For this review, use the dimensioned drawing (mm, ordinates from the lowest corner) and the shaded views. A direction names the side the tool comes from. Round coordinates to 2 decimals unless told otherwise and drop trailing zeros. Loops run counter-clockwise (first coordinate to the right, second up) from the corner with the lowest first, then second, coordinate; pieces in that order, holes last. Notation, with made-up numbers: M -39.75,-37 L -14.75,-37 A20 ccw -14.75,-11 Z; hole C 64,68 d10. An arc over 180 degrees is marked long. One line per item, written item: value. Start each with the question number.
Item 1: For the marked faces 1 and 2, list the 3-axis set-ups (+Z, -Z, +X, -X, +Y, -Y) from which the entire face can be reached by the end or side of a thin tool; tool diameter is ignored.
Item 2: We need section A-A (y = 12.5). Write out the cut boundary in (x, z), then the cut area to 3 significant figures.
Item 3: For line 1 along Z through (x, y) = (10.25, 12.75); line 2 along Z through (x, y) = (12.5, 20.5); line 3 along X through (y, z) = (17.5, 8.5), list the stretches that pass through material, from the lowest coordinate up.
Item 4: We need section C-C (z = 13.5). Write out the cut boundary in (x, y).
Item 5: We need section B-B (z = 31). Write out the cut boundary in (x, y).
Item 6: Clearance check with flat-ended pins moving along their axes: pin 1 (5 mm diameter, centred on x = 16.5, z = 6.5, fed in from -Y); pin 2 (1.5 mm diameter, centred on x = 13.5, z = 9.5, fed in from -Y); pin 3 (5 mm diameter, centred on x = 8, z = 17.5, fed in from +Y). State where each tip first meets the part, or that it passes through.
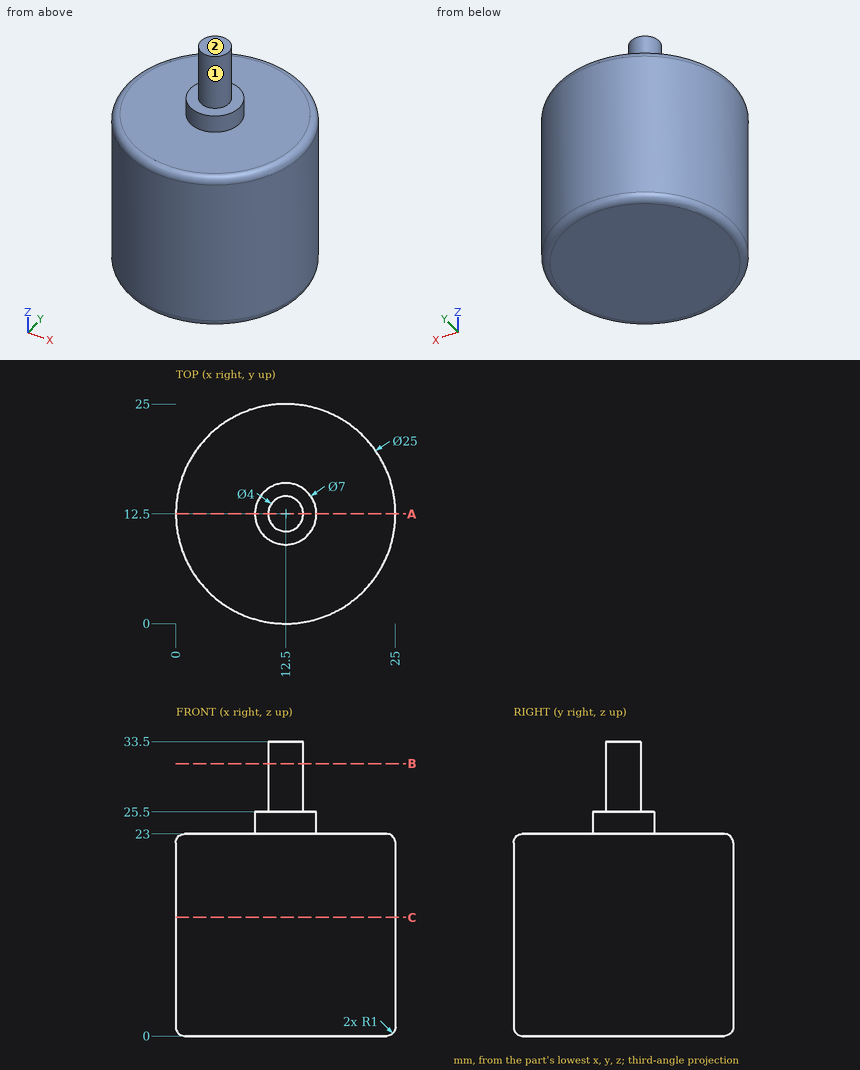
A:
1. face 1: +Z
1. face 2: +Z, +X, -X, +Y, -Y
2. outline: M 0,1 A1 ccw 1,0 L 24,0 A1 ccw 25,1 L 25,22 A1 ccw 24,23 L 16,23 L 16,25.5 L 14.5,25.5 L 14.5,33.5 L 10.5,33.5 L 10.5,25.5 L 9,25.5 L 9,23 L 1,23 A1 ccw 0,22 Z
2. area: 624 mm2
3. line 1: 0 to 25.5
3. line 2: 0 to 23
3. line 3: 1.04 to 23.96
4. outline: C 12.5,12.5 d25
5. outline: C 12.5,12.5 d4
6. pin 1: y = 0.09
6. pin 2: y = 0
6. pin 3: y = 24.84
